```python
from build123d import *

# Parameters (mm, degrees)
SKETCH1_W            = 7
SKETCH1_H            = 18
BOSS_EXTRUDE1_DEPTH  = 8
SKETCH3_W            = 7
SKETCH3_H            = 18
BOSS_EXTRUDE2_DEPTH  = 2
SKETCH2_W            = 5
SKETCH2_H            = 5.5
CUT_EXTRUDE1_DEPTH   = 8
SKETCH4_R            = 1
CUT_EXTRUDE2_DEPTH   = 3
SKETCH5_W            = 5
SKETCH5_H            = 10
BOSS_EXTRUDE3_DEPTH  = 3
FILLET1_R            = 2
FILLET1_OF_MIRROR2_R = 2
FILLET2_R            = 1


with BuildPart() as part:
    # Sketch1 → Boss-Extrude1 (new body)
    with BuildSketch(Plane.XY):
        Rectangle(SKETCH1_W, SKETCH1_H)
    extrude(amount=BOSS_EXTRUDE1_DEPTH)

    # Sketch3 → Boss-Extrude2 (add)
    with BuildSketch(Plane(origin=(0, 0, 0), x_dir=(-1, 0, 0), z_dir=(0, 0, -1))):
        Rectangle(SKETCH3_W, SKETCH3_H)
    extrude(amount=BOSS_EXTRUDE2_DEPTH)

    # Sketch2 → Cut-Extrude1 (cut)
    with BuildSketch(Plane.XY.offset(8)):
        with Locations((0, 4.33)):
            Rectangle(SKETCH2_W, SKETCH2_H)
        with Locations((0, -3.02)):
            Rectangle(SKETCH2_W, SKETCH2_H)
    extrude(amount=-CUT_EXTRUDE1_DEPTH, mode=Mode.SUBTRACT)

    # Sketch4 → Cut-Extrude2 (cut, through all)
    with BuildSketch(Plane.XY):
        with Locations((0, 4.33)):
            Circle(SKETCH4_R)
        with Locations((0, -3.02)):
            Circle(SKETCH4_R)
    extrude(amount=-CUT_EXTRUDE2_DEPTH, mode=Mode.SUBTRACT)

    # Sketch5 → Boss-Extrude3 (add)
    with BuildSketch(Plane.XZ.offset(9)):
        with Locations((6, 3)):
            Rectangle(SKETCH5_W, SKETCH5_H)
        with BuildLine():
            Line((7.5, 4.5), (7.5, 1.5))
            ThreePointArc((7.5, 1.5), (6, 0), (4.5, 1.5))
            Line((4.5, 1.5), (4.5, 4.5))
            ThreePointArc((4.5, 4.5), (6, 6), (7.5, 4.5))
        make_face(mode=Mode.SUBTRACT)
    boss_extrude3 = extrude(amount=-BOSS_EXTRUDE3_DEPTH)

    # Fillet1
    fillet1_edges = [part.edges().sort_by_distance(p)[0] for p in [
        (8.5, -7.5, -2),
        (8.5, -7.5, 8),
    ]]
    fillet(fillet1_edges, radius=FILLET1_R)

    # Mirror2: Boss-Extrude3 across plane
    add(boss_extrude3.mirror(Plane(origin=(0, 0, 0), x_dir=(0, 0, 1), z_dir=(1, 0, 0))))

    # Fillet1 of Mirror2
    fillet1_of_mirror2_edges = [part.edges().sort_by_distance(p)[0] for p in [
        (-8.5, -7.5, -2),
        (-8.5, -7.5, 8),
    ]]
    fillet(fillet1_of_mirror2_edges, radius=FILLET1_OF_MIRROR2_R)

    # Fillet2
    fillet2_edges = [part.edges().sort_by_distance(p)[0] for p in [
        (3.5, 9, 3),
        (-3.5, 9, 3),
    ]]
    fillet(fillet2_edges, radius=FILLET2_R)


solid = part.part
```
Check sheet for the modelled part. Datum: model origin and axes. Units: mm. A direction names the side the tool comes from. Give positions to 0.01 mm unless a question says otherwise; leave off trailing zeros. Write each loop counter-clockwise with the first axis right and the second up, starting at its lowest first coordinate (ties: lowest second). Pieces come first, ordered by that corner, then holes. Notation, with made-up numbers: (86.25, -12) - (115.25, -12) arc R10 cw to (115.25, 4) - close; hole circle Ø2 at (69, 9.25). An arc over 180 degrees is marked (long way). Answer as a JSON object with one key per item and string values. Group by question number.
1) Sectioned sample at C-C (x = -6). Record the cut outline in (y, z), then the cut area to 3 significant figures.
2) Release check for a two-part mould opening along Z. For faces 4 (the face through (0, -9, 3)), 5 (the face through (-1.15, 4.37, 0)), 6 (the face through (-6, -8, 6)), 7 (the face through (-6, -8, 0)) record: pulls with the +Z half, pulls with the -Z half, needs draft (parallel to the pull), parting line crosses it, or undercut.
3) Sectioned sample at A-A (y = -3.02). Record the cut outline in (x, z), then the cut area to 3 significant figures.
4) Access from +Z, -Z, +X, -X, +Y, -Y to the whole of each face (thin tool, end or side, straight path). Record for faces 1 (the face through (-3.5, 1, 3)), 2 (the face through (-2.5, -3, 4)), 3 (the face through (-4.5, -8, 3)).
5) Depth check by flat-ended pin: P1, Ø6, axis at y = -2.5, z = 3, coming from the -X side; P2, Ø1, axis at x = 5, y = 2, coming from the -Z side; P3, Ø4.5, axis at y = 3.5, z = 2.5, coming from the +X side; P4, Ø2.5, axis at x = 0, y = 4.33, coming from the +Z side. Enter the tip coordinate at first touch or a pass-through.
6) Sectioned sample at B-B (z = 1.25). Record the cut outline in (x, y), then the cut area to 3 significant figures.
7) Sectioned sample at D-D (y = 5.75). Record the cut outline in (x, z).
8) Thickness scan on probe 1 along Y at (x, z) = (0, -0.95); probe 2 along X at (y, z) = (-3.25, 7.5); probe 3 along X at (y, z) = (1.5, -1.5). Record the ranges inside material, lowest first. Write a range as from..to.
Geometry results:
{
 "1": {"outline": "(-9, -2) - (-6, -2) - (-6, 0) - (-9, 0) - close; (-9, 6) - (-6, 6) - (-6, 8) - (-9, 8) - close", "area": "12.0 mm^2"},
 "2": {"face 4": "needs draft", "face 5": "pulls with the +Z half", "face 6": "undercut", "face 7": "undercut"},
 "3": {"outline": "(-3.5, -2) - (-1, -2) - (-1, 0) - (-2.5, 0) - (-2.5, 8) - (-3.5, 8) - close; (1, -2) - (3.5, -2) - (3.5, 8) - (2.5, 8) - (2.5, 0) - (1, 0) - close", "area": "26.0 mm^2"},
 "4": {"face 1": "+Z, -Z, -X, +Y", "face 2": "+Z", "face 3": "+Y, -Y"},
 "5": {"P1": "stops at x = -3.5", "P2": "passes through", "P3": "stops at x = 3.5", "P4": "stops at z = 0"},
 "6": {"outline": "(-8.5, -9) - (-7.48, -9) - (-7.48, -6) - (-8.5, -6) - close; (-4.52, -9) - (4.52, -9) - (4.52, -6) - (3.5, -6) - (3.5, 8) arc R1 ccw to (2.5, 9) - (-2.5, 9) arc R1 ccw to (-3.5, 8) - (-3.5, -6) - (-4.52, -6) - close; (7.48, -9) - (8.5, -9) - (8.5, -6) - (7.48, -6) - close; hole (-2.5, -5.77) - (2.5, -5.77) - (2.5, -0.27) - (-2.5, -0.27) - close; hole (-2.5, 1.58) - (2.5, 1.58) - (2.5, 7.08) - (-2.5, 7.08) - close", "area": "82.8 mm^2"},
 "7": {"outline": "(-3.5, -2) - (3.5, -2) - (3.5, 8) - (2.5, 8) - (2.5, 0) - (-2.5, 0) - (-2.5, 8) - (-3.5, 8) - close"},
 "8": {"probe 1": "y = -9..-4.02, -2.02..3.33, 5.33..9", "probe 2": "x = -3.5..-2.5, 2.5..3.5", "probe 3": "x = -3.5..3.5"}
}
